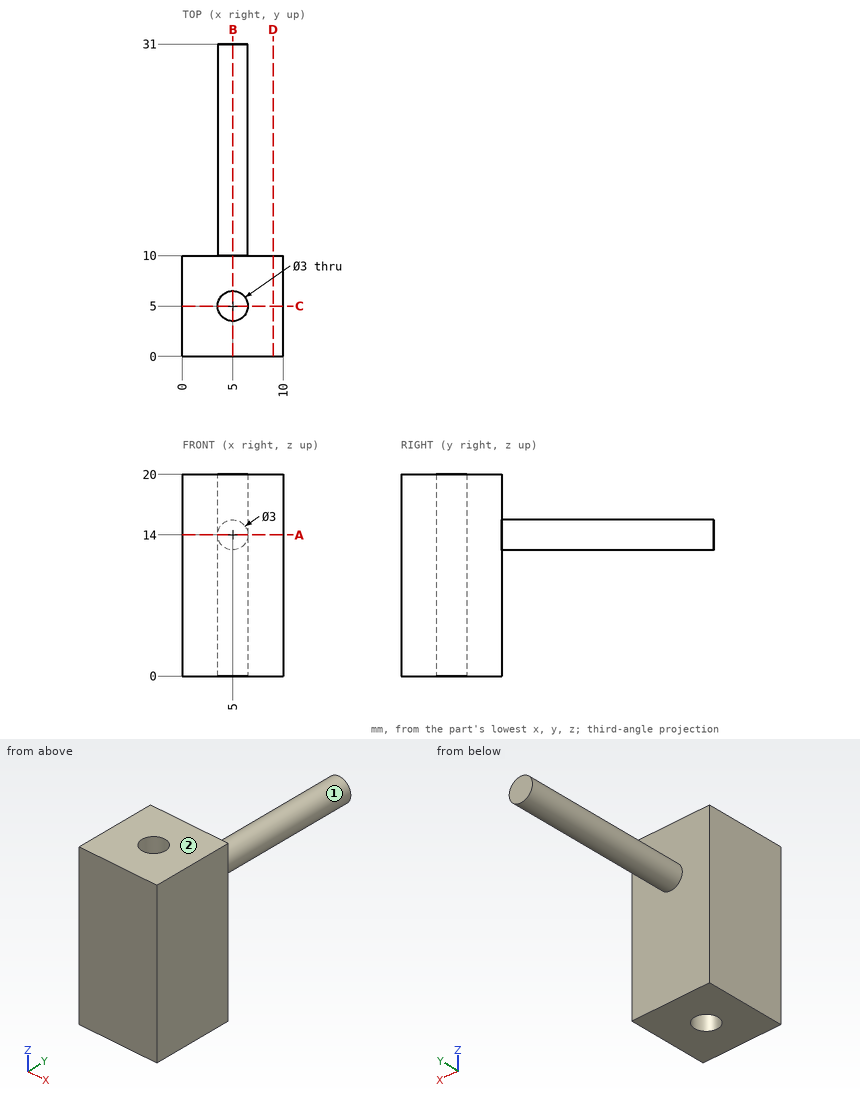
Here's the drawing with two shaded views (mm, measured from the low corner). I have some questions. A direction names the side the tool comes from. Round coordinates to 2 decimals unless told otherwise and drop trailing zeros. Order: outer loops, then holes, each group sorted by start corner. A loop starts at its lowest first (then second) coordinate and runs counter-clockwise, first axis right, second up. Notation, with made-up numbers: M 67,81 L 85,81 A20 ccw 85,105 Z; hole C 84,66.5 d4. An arc over 180 degrees is marked long. Answer in a Markdown table with one row per item.
Item 1: I'm going to push flat-ended pins straight in: pin 1 (1.5 mm diameter, centred on x = 4, y = 4, fed in from +Z); pin 2 (1 mm diameter, centred on x = 4.5, y = 27, fed in from -Z); pin 3 (1 mm diameter, centred on y = 22.5, z = 17.5, fed in from +X); pin 4 (3 mm diameter, centred on y = 23, z = 16.5, fed in from +X). Where does each tip first touch, or does it pass through?
A:
| item | result |
|---|---|
| pin 1 | stops at z = 20 |
| pin 2 | stops at z = 12.5 |
| pin 3 | passes through |
| pin 4 | stops at x = 6.12 |
Item 2: Imagine slicing it at B-B, the plane x = 5. Write out the boundary of the cut face in (y, z).
A:
| item | result |
|---|---|
| outline | M 0,0 L 3.5,0 L 3.5,20 L 0,20 Z; M 6.5,0 L 10,0 L 10,12.5 L 31,12.5 L 31,15.5 L 10,15.5 L 10,20 L 6.5,20 Z |
Item 3: If I drill on L1, parallel to Y at x = 5, z = 11.75; L2, parallel to Y at x = 4, z = 13; L3, parallel to Z at x = 4, y = 19, over which ranges is the centre line in solid material (lowest first)? Write a range as from..to.
A:
| item | result |
|---|---|
| L1 | y = 0..3.5, 6.5..10 |
| L2 | y = 0..3.88, 6.12..31 |
| L3 | z = 12.88..15.12 |
Item 4: Imagine slicing it at C-C, the plane y = 5. Write out the boundary of the cut face in (x, z), and give its area (3 significant figures).
A:
| item | result |
|---|---|
| outline | M 0,0 L 3.5,0 L 3.5,20 L 0,20 Z; M 6.5,0 L 10,0 L 10,20 L 6.5,20 Z |
| area | 140 mm2 |
Item 5: Imagine slicing it at A-A, the plane z = 14. Write out the boundary of the cut face in (x, y), and give its area (3 significant figures).
A:
| item | result |
|---|---|
| outline | M 0,0 L 10,0 L 10,10 L 6.5,10 L 6.5,31 L 3.5,31 L 3.5,10 L 0,10 Z; hole C 5,5 d3 |
| area | 156 mm2 |
Item 6: For the marked faces 1 and 2, which set-ups out of +Z, -Z, +X, -X, +Y, -Y let a thin tool reach every point of the face, with its end or its side?
A:
| item | result |
|---|---|
| face 1 | +Y |
| face 2 | +Z, +X, -X, +Y, -Y |
Item 7: Imagine slicing it at D-D, the plane x = 9. Write out the boundary of the cut face in (y, z), and give its area (3 significant figures).
A:
| item | result |
|---|---|
| outline | M 0,0 L 10,0 L 10,20 L 0,20 Z |
| area | 200 mm2 |
